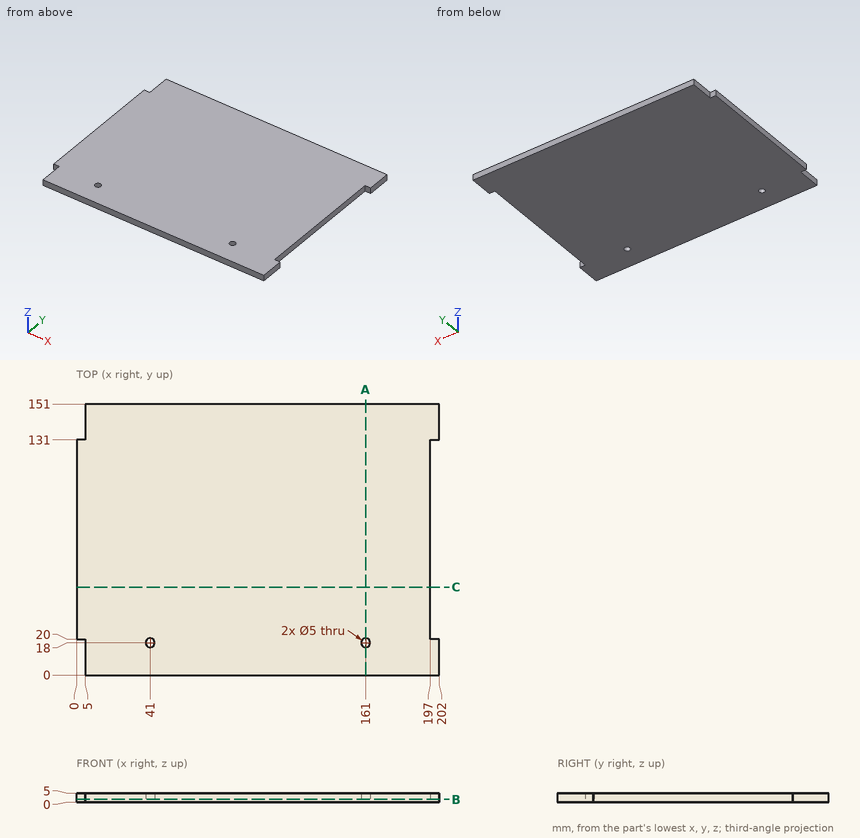
Source: three-view drawing plus pictorial views. Frame: mm from the lowest corner of the part. Give positions to 0.01 mm unless a question says otherwise; leave off trailing zeros. Order: outer loops, then holes, each group sorted by start corner. A loop starts at its lowest first (then second) coordinate and runs counter-clockwise, first axis right, second up.
1. Pin query (flat end, axial travel): pin 1 (1.5 mm diameter, centred on y = 88.5, z = 3.5, fed in from +X); pin 2 (3 mm diameter, centred on x = 161, y = 18, fed in from -Z); pin 3 (2.5 mm diameter, centred on y = 141.5, z = 3.5, fed in from -X); pin 4 (1.5 mm diameter, centred on x = 1.5, z = 3, fed in from +Y). Return the tip coordinate at first contact, or that it passes through.
Derived:
pin 1: stops at x = 197
pin 2: passes through
pin 3: stops at x = 5
pin 4: stops at y = 131
2. Section C-C on y = 49. Return the cut outline in (x, z).
Derived:
outline: (0, 0) - (197, 0) - (197, 5) - (0, 5) - close
3. Material intervals for L1, parallel to Y at x = 41, z = 2.35; L2, parallel to X at y = 69, z = 2.95; L3, parallel to Y at x = 160, z = 4.5, sorted ascending.
Derived:
L1: y = 0 to 15.5, 20.5 to 151
L2: x = 0 to 197
L3: y = 0 to 15.71, 20.29 to 151
4. Section B-B on z = 1.55. Return the cut outline in (x, y).
Derived:
outline: (0, 20) - (5, 20) - (5, 0) - (202, 0) - (202, 20) - (197, 20) - (197, 131) - (202, 131) - (202, 151) - (5, 151) - (5, 131) - (0, 131) - close; hole circle Ø5 at (41, 18); hole circle Ø5 at (161, 18)
5. Section A-A on x = 161. Return the cut outline in (y, z).
Derived:
outline: (0, 0) - (15.5, 0) - (15.5, 5) - (0, 5) - close; (20.5, 0) - (151, 0) - (151, 5) - (20.5, 5) - close
